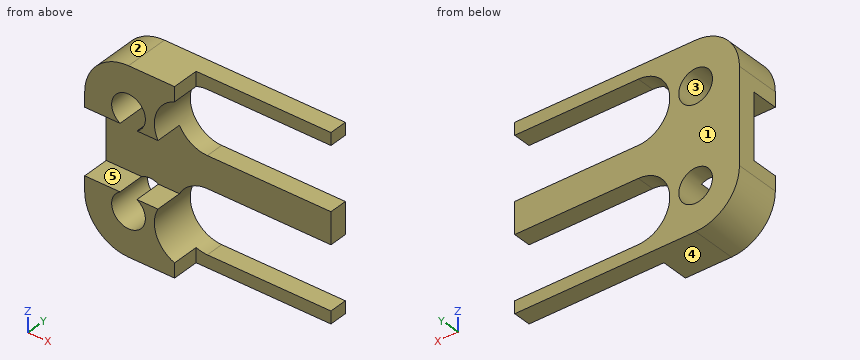
from build123d import *

# Parameters (mm, degrees)
CROQUIS1_R              = 3.75
SALIENTE_EXTRUIR1_DEPTH = 10
CROQUIS2_W              = 40.5
CROQUIS2_H              = 4
SALIENTE_EXTRUIR2_DEPTH = 30
CROQUIS3_W              = 14.5
CROQUIS3_H              = 6
CORTAR_EXTRUIR1_DEPTH   = 38.550798926
CORTAR_EXTRUIR2_DEPTH   = 47.15327724


with BuildPart() as part:
    # Croquis1 → Saliente-Extruir1 (new body)
    with BuildSketch(Plane(origin=(0, 0, 0), x_dir=(1, 0, 0), z_dir=(0, 1, 0))):
        with BuildLine():
            Line((-9.75, -10.5), (-9.75, 10.5))
            ThreePointArc((-9.75, 10.5), (-6.894291117, 17.394291117), (0, 20.25))
            Line((0, 20.25), (10.25, 20.25))
            Line((10.25, 20.25), (10.25, -20.25))
            Line((10.25, -20.25), (0, -20.25))
            ThreePointArc((0, -20.25), (-6.894291117, -17.394291117), (-9.75, -10.5))
        make_face()
        with Locations(Location((0, 10.5, 0), (0, 0, 270))):
            Circle(CROQUIS1_R, mode=Mode.SUBTRACT)
        with Locations(Location((0, -10.5, 0), (0, 0, 270))):
            Circle(CROQUIS1_R, mode=Mode.SUBTRACT)
    extrude(amount=SALIENTE_EXTRUIR1_DEPTH)

    # Croquis2 → Saliente-Extruir2 (add)
    with BuildSketch(Plane(origin=(10.25, 0, 0), x_dir=(0, 0, -1), z_dir=(1, 0, 0))):
        with Locations((0, 8)):
            Rectangle(CROQUIS2_W, CROQUIS2_H)
    extrude(amount=SALIENTE_EXTRUIR2_DEPTH)

    # Croquis3 → Cortar-Extruir1 (cut, through all)
    with BuildSketch(Plane(origin=(10.25, 0, 0), x_dir=(0, 0, -1), z_dir=(1, 0, 0))):
        with Locations((0, 3)):
            Rectangle(CROQUIS3_W, CROQUIS3_H)
    extrude(amount=-CORTAR_EXTRUIR1_DEPTH, mode=Mode.SUBTRACT)

    # Croquis5 → Cortar-Extruir2 (cut, through all)
    with BuildSketch(Plane(origin=(0, 10, 0), x_dir=(1, 0, 0), z_dir=(0, 1, 0))):
        with BuildLine():
            Line((12.75, -3.5), (40.25, -3.5))
            ThreePointArc((40.25, -3.5), (47.25, -10.5), (40.25, -17.5))
            Line((40.25, -17.5), (12.75, -17.5))
            ThreePointArc((12.75, -17.5), (5.75, -10.5), (12.75, -3.5))
        make_face()
        with BuildLine():
            Line((12.75, 3.5), (40.25, 3.5))
            ThreePointArc((40.25, 3.5), (47.25, 10.5), (40.25, 17.5))
            Line((40.25, 17.5), (12.75, 17.5))
            ThreePointArc((12.75, 17.5), (5.75, 10.5), (12.75, 3.5))
        make_face()
    extrude(amount=-CORTAR_EXTRUIR2_DEPTH, mode=Mode.SUBTRACT)


solid = part.part
Check sheet for the modelled part. Datum: model origin and axes. Units: mm. Face numbers are marked on the shaded views. A direction names the side the tool comes from. Round coordinates to 2 decimals unless told otherwise and drop trailing zeros. Loops run counter-clockwise (first coordinate to the right, second up) from the corner with the lowest first, then second, coordinate; pieces in that order, holes last.
1. Set-up check for the marked faces 4 and 5: record each of +Z, -Z, +X, -X, +Y, -Y from which the full face is reachable in a straight line by a thin tool's end or side.
2. Sectioned sample at A-A on x = 21.5. Record the boundary of the cut face in (y, z), and give its area (3 significant figures).
3. Mould release check, pull along Z, two halves, no side actions. Record for the marked faces 1, 2 and 3: released by +Z, released by -Z, zero draft, split by the parting line, or undercut.
4. Sectioned sample at C-C on z = -9.5. Record the boundary of the cut face in (x, y), and give its area (3 significant figures).
5. Gauge pin test, flat ends, axial feed: pin 1 Ø7 at (x, z) = (26.5, -2) entering from -Y; pin 2 Ø2.5 at (y, z) = (4.5, -19.5) entering from +X; pin 3 Ø5 at (x, y) = (-4, 1.5) entering from +Z. Record the tip position at first contact, or that the pin passes through.
6. Sectioned sample at B-B on y = 2. Record the boundary of the cut face in (x, z).
7. Sectioned sample at D-D on y = 7.75. Record the boundary of the cut face in (x, z), and give its area (3 significant figures).
8. Scan lines: probe 1 along Z at (x, y) = (26.5, 8); probe 2 along X at (y, z) = (6, 10.5). Record each from-to range of solid material in increasing order.
Recorded:
1. face 4: -Z, +X, -X, +Y, -Y
1. face 5: +X, -X, -Y
2. outline: (6, -20.25) - (10, -20.25) - (10, -17.5) - (6, -17.5) - close; (6, -3.5) - (10, -3.5) - (10, 3.5) - (6, 3.5) - close; (6, 17.5) - (10, 17.5) - (10, 20.25) - (6, 20.25) - close
2. area: 50.0 mm2
3. face 1: zero draft
3. face 2: released by +Z
3. face 3: undercut
4. outline: (-9.75, 0) - (-3.61, 0) - (-3.61, 10) - (-9.75, 10) - close; (3.61, 0) - (5.82, 0) - (5.82, 10) - (3.61, 10) - close
4. area: 83.4 mm2
5. pin 1: stops at y = 6
5. pin 2: stops at x = 10.25
5. pin 3: stops at z = 20.13
6. outline: (-9.75, -10.5) arc R9.75 ccw to (0, -20.25) - (10.25, -20.25) - (10.25, -17.04) arc R7 cw to (6.55, -7.25) - (1.87, -7.25) arc R3.75 cw (long way) to (-1.87, -7.25) - (-9.75, -7.25) - close; (-9.75, 7.25) - (-1.87, 7.25) arc R3.75 cw (long way) to (1.87, 7.25) - (6.55, 7.25) arc R7 cw to (10.25, 17.04) - (10.25, 20.25) - (0, 20.25) arc R9.75 ccw to (-9.75, 10.5) - close
7. outline: (-9.75, -10.5) arc R9.75 ccw to (0, -20.25) - (40.25, -20.25) - (40.25, -17.5) - (12.75, -17.5) arc R7 cw to (12.75, -3.5) - (40.25, -3.5) - (40.25, 3.5) - (12.75, 3.5) arc R7 cw to (12.75, 17.5) - (40.25, 17.5) - (40.25, 20.25) - (0, 20.25) arc R9.75 ccw to (-9.75, 10.5) - close; hole circle Ø7.5 at (0, -10.5); hole circle Ø7.5 at (0, 10.5)
7. area: 972 mm2
8. probe 1: z = -20.25 to -17.5, -3.5 to 3.5, 17.5 to 20.25
8. probe 2: x = -9.75 to -3.75, 3.75 to 5.75
